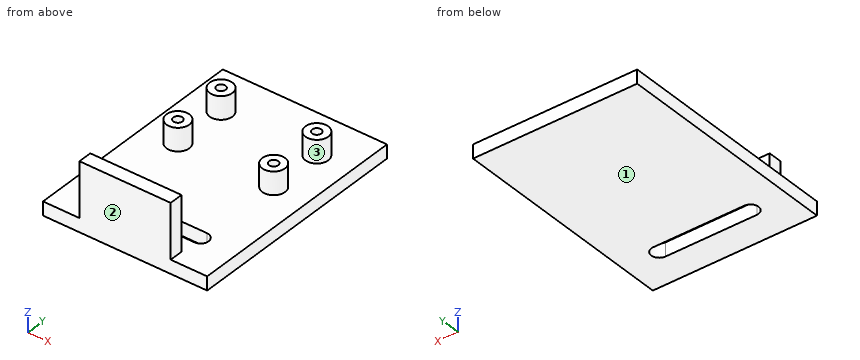
from build123d import *

# Parameters (mm, degrees)
SKETCH1_W           = 36
SKETCH1_H           = 50
BOSS_EXTRUDE1_DEPTH = 3
SKETCH2_W           = 20
SKETCH2_H           = 3
BOSS_EXTRUDE2_DEPTH = 12
CUT_EXTRUDE1_DEPTH  = 5
SKETCH5_R           = 2.5
SKETCH5_R_2         = 1
BOSS_EXTRUDE4_DEPTH = 5


with BuildPart() as part:
    # Sketch1 → Boss-Extrude1 (new body)
    with BuildSketch(Plane.XY):
        with Locations((-6.367052023, -5.057803468)):
            Rectangle(SKETCH1_W, SKETCH1_H)
    extrude(amount=BOSS_EXTRUDE1_DEPTH)

    # Sketch2 → Boss-Extrude2 (add)
    with BuildSketch(Plane.XY.offset(3)):
        with Locations((-6.367052023, -28.557803468)):
            Rectangle(SKETCH2_W, SKETCH2_H)
    extrude(amount=BOSS_EXTRUDE2_DEPTH)

    # Sketch4 → Cut-Extrude1 (cut)
    with BuildSketch(Plane.XY.offset(3)):
        with BuildLine():
            Line((-16.367052023, -19.980355704), (3.632947977, -19.980355704))
            ThreePointArc((3.632947977, -19.980355704), (5.373912404, -21.721320132), (3.632947977, -23.462284559))
            Line((3.632947977, -23.462284559), (-16.367052023, -23.462284559))
            ThreePointArc((-16.367052023, -23.462284559), (-18.108016451, -21.721320132), (-16.367052023, -19.980355704))
        make_face()
    extrude(amount=-CUT_EXTRUDE1_DEPTH, mode=Mode.SUBTRACT)

    # Sketch5 → Boss-Extrude4 (add)
    # profile 1 of 4: a face of its own
    with BuildSketch(Plane.XY.offset(3)):
        with Locations(Location((4.132947977, 9.942196532, 0), (0, 0, 180))):
            Circle(SKETCH5_R)
        with Locations((4.132947977, 9.942196532)):
            Circle(SKETCH5_R_2, mode=Mode.SUBTRACT)
    # profile 2 of 4: a face of its own
    with BuildSketch(Plane.XY.offset(3)):
        with Locations(Location((-16.867052023, 9.942196532, 0), (0, 0, 180))):
            Circle(SKETCH5_R)
        with Locations((-16.867052023, 9.942196532)):
            Circle(SKETCH5_R_2, mode=Mode.SUBTRACT)
    # profile 3 of 4: a face of its own
    with BuildSketch(Plane.XY.offset(3)):
        with Locations(Location((-16.867052023, -2.057803468, 0), (0, 0, 180))):
            Circle(SKETCH5_R)
        with Locations((-16.867052023, -2.057803468)):
            Circle(SKETCH5_R_2, mode=Mode.SUBTRACT)
    # profile 4 of 4: a face of its own
    with BuildSketch(Plane.XY.offset(3)):
        with Locations(Location((4.132947977, -2.057803468, 0), (0, 0, 180))):
            Circle(SKETCH5_R)
        with Locations((4.132947977, -2.057803468)):
            Circle(SKETCH5_R_2, mode=Mode.SUBTRACT)
    extrude(amount=BOSS_EXTRUDE4_DEPTH)


solid = part.part
Geometry: final body of the model. Coordinates: model frame, mm. Face numbers are marked on the shaded views. Coordinates: 2 decimals unless noted, no trailing zeros. Write each loop counter-clockwise with the first axis right and the second up, starting at its lowest first coordinate (ties: lowest second). Pieces come first, ordered by that corner, then holes. Notation, with made-up numbers: (-30, 22) - (-25, 22) arc R36 ccw to (-25, 59) - close; hole circle Ø10 at (66.25, 28.25). An arc over 180 degrees is marked (long way). Return JSON: item names as keys, results as strings.
Item 1: Section query D-D (y = -12). Output: boundary loops of the cut face in (x, z).
Completed:
{"outline": "(-24.37, 0) - (11.63, 0) - (11.63, 3) - (-24.37, 3) - close"}
Item 2: Section query A-A (x = -10). Output: boundary loops of the cut face in (y, z).
Completed:
{"outline": "(-30.06, 0) - (-23.46, 0) - (-23.46, 3) - (-27.06, 3) - (-27.06, 15) - (-30.06, 15) - close; (-19.98, 0) - (19.94, 0) - (19.94, 3) - (-19.98, 3) - close"}
Item 3: Section query C-C (z = 2). Output: boundary loops of the cut face in (x, y).
Completed:
{"outline": "(-24.37, -30.06) - (11.63, -30.06) - (11.63, 19.94) - (-24.37, 19.94) - close; hole (-16.37, -23.46) - (3.63, -23.46) arc R1.74 ccw to (3.63, -19.98) - (-16.37, -19.98) arc R1.74 ccw to start"}
Item 4: Section query B-B (z = 7.25). Count the separate pieces of the cut face and the enclosed holes in it, and give its area (3 significant figures).
Completed:
{"separate pieces": "5", "enclosed holes": "4", "area": "126 mm2"}
Item 5: Line query: L1, parallel to Y at x = -17, z = 5.5; L2, parallel to Y at x = -2, z = 8.25; L3, parallel to Z at x = 9.5, y = -13. Output: solid intervals per line, ascending.
Completed:
{"L1": "y = -4.55 to -3.05, -1.07 to 0.44, 7.45 to 8.95, 10.93 to 12.44", "L2": "y = -30.06 to -27.06", "L3": "z = 0 to 3"}
Item 6: Pull-direction query (Y, two-part tool) for the marked faces 1, 2 and 3; classes: +Y half, -Y half, draft (parallel to the pull), parting line (faces both ways), or undercut.
Completed:
{"face 1": "draft", "face 2": "-Y half", "face 3": "undercut"}
Item 7: Pin query (flat end, axial travel): pin 1 Ø8 at (y, z) = (-13, 9) entering from +X; pin 2 Ø1.5 at (x, y) = (-17.5, -1) entering from +Z; pin 3 Ø1.5 at (y, z) = (-28.5, 7) entering from -X; pin 4 Ø1 at (x, y) = (-7.5, 11.5) entering from +Z. Return the tip coordinate at first contact, or that it passes through.
Completed:
{"pin 1": "passes through", "pin 2": "stops at z = 8", "pin 3": "stops at x = -16.37", "pin 4": "stops at z = 3"}
